Verification items for the finished model (mm, model axes). Face numbers are marked on the shaded views. A direction names the side the tool comes from. Round coordinates to 2 decimals unless told otherwise and drop trailing zeros. Order: outer loops, then holes, each group sorted by start corner. A loop starts at its lowest first (then second) coordinate and runs counter-clockwise, first axis right, second up. Notation, with made-up numbers: (69.25, -16.5) -> (100.25, -16.5) arc R25 cw to (100.25, 4.5) -> close; hole circle Ø4 at (39.25, 88.5). An arc over 180 degrees is marked (long way). Put each result on its own line as item: value.
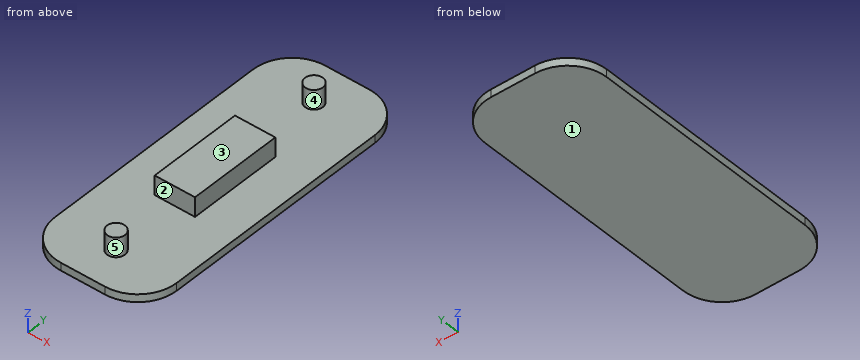
from build123d import *

# Parameters (mm, degrees)
F0_W     = 31.366382
F0_H     = 80
F1_DEPTH = 2
F2_W     = 10.4
F2_H     = 24.3
F2_R     = 2.3
F3_DEPTH = 5
F4_R     = 10


with BuildPart() as f1:
    # F0 (on Top) → F1 (new body)
    with BuildSketch(Plane.XY):
        Rectangle(F0_W, F0_H)
    extrude(amount=F1_DEPTH)

    # F2 (on face) → F3 (join)
    with BuildSketch(Plane.XY.offset(2)):
        Rectangle(F2_W, F2_H)
        with Locations((0, 29.95)):
            Circle(F2_R)
        with Locations((0, -29.95)):
            Circle(F2_R)
    extrude(amount=F3_DEPTH)

    # F4
    f4_edges = [f1.edges().sort_by_distance(p)[0] for p in [
        (-15.683191, 40, 1),
        (15.683191, 40, 1),
        (15.683191, -40, 1),
        (-15.683191, -40, 1),
    ]]
    fillet(f4_edges, radius=F4_R)


solid = f1.part
Item 1: Tool access check on the marked faces 1 and 2. Record the directions out of +Z, -Z, +X, -X, +Y, -Y that give a thin tool (end or side, any length) a straight path to the whole face; none if there is none.
Check sheet entries:
face 1: -Z, +X, -X, +Y, -Y
face 2: +Z, +X, -X
Item 2: Section check C-C on y = 8.5. Record the boundary of the cut face in (x, z), then the cut area to 3 significant figures.
Check sheet entries:
outline: (-15.68, 0) -> (15.68, 0) -> (15.68, 2) -> (5.2, 2) -> (5.2, 7) -> (-5.2, 7) -> (-5.2, 2) -> (-15.68, 2) -> close
area: 115 mm^2
Item 3: Section check D-D on y = -24.5. Record the boundary of the cut face in (x, z).
Check sheet entries:
outline: (-15.68, 0) -> (15.68, 0) -> (15.68, 2) -> (-15.68, 2) -> close
Item 4: Release check for a two-part mould opening along Y. For the marked faces 3, 4 and 5 record: +Y half, -Y half, draft (parallel to the pull), parting line (faces both ways), or undercut.
Check sheet entries:
face 3: draft
face 4: undercut
face 5: undercut
Item 5: Material ranges on L1, parallel to Y at x = -2, z = 6; L2, parallel to Z at x = 10, y = -24; L3, parallel to Y at x = -4, z = 6.25, recorded low to high. Write a range as [from, to].
Check sheet entries:
L1: y = [-31.09, -28.81], [-12.15, 12.15], [28.81, 31.09]
L2: z = [0, 2]
L3: y = [-12.15, 12.15]
Item 6: Section check A-A on x = 0. Record the boundary of the cut face in (y, z).
Check sheet entries:
outline: (-40, 0) -> (40, 0) -> (40, 2) -> (32.25, 2) -> (32.25, 7) -> (27.65, 7) -> (27.65, 2) -> (12.15, 2) -> (12.15, 7) -> (-12.15, 7) -> (-12.15, 2) -> (-27.65, 2) -> (-27.65, 7) -> (-32.25, 7) -> (-32.25, 2) -> (-40, 2) -> close
Item 7: Gauge pin test, flat ends, axial feed: pin 1 Ø2.5 at (y, z) = (-2, 4) entering from -X; pin 2 Ø6 at (x, y) = (-7, 24.5) entering from +Z; pin 3 Ø1.5 at (y, z) = (-4, 4) entering from +X. Record the tip position at first contact, or that the pin passes through.
Check sheet entries:
pin 1: stops at x = -5.2
pin 2: stops at z = 2
pin 3: stops at x = 5.2
Item 8: Section check B-B on z = 3.75. Record the boundary of the cut face in (x, y).
Check sheet entries:
outline: (-5.2, -12.15) -> (5.2, -12.15) -> (5.2, 12.15) -> (-5.2, 12.15) -> close; circle Ø4.6 at (0, -29.95); circle Ø4.6 at (0, 29.95)
